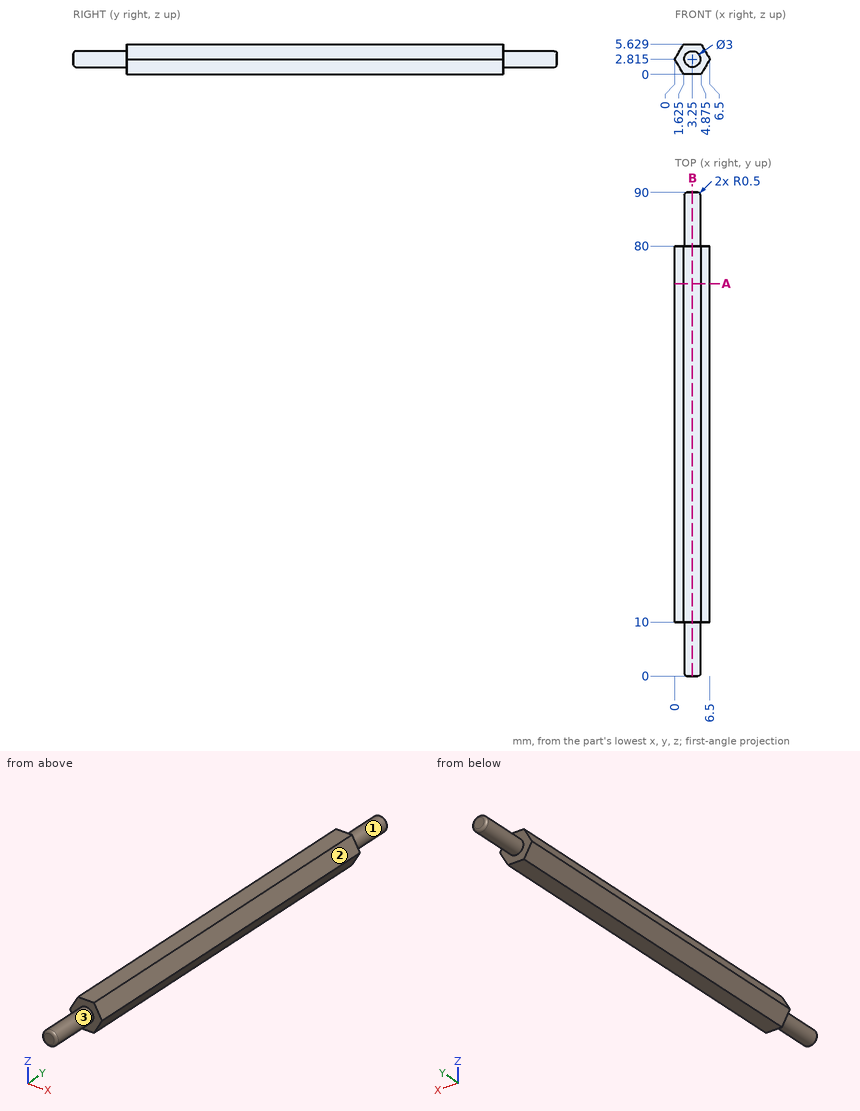
Geometry check sheet. Reference: drawing and pictorial views, mm from the part's lowest x, y, z. A direction names the side the tool comes from. Round coordinates to 2 decimals unless told otherwise and drop trailing zeros. Order: outer loops, then holes, each group sorted by start corner. A loop starts at its lowest first (then second) coordinate and runs counter-clockwise, first axis right, second up. Notation, with made-up numbers: (-11, 17.25) - (11, 17.25) arc R5 cw to (11, 26.25) - close; hole circle Ø2 at (80, 31). An arc over 180 degrees is marked (long way). Use a Markdown table: item, result. Add a question column.
1) Section check B-B (x = 3.25). Record the cut outline in (y, z) (1 decimal).
2) Section check A-A (y = 73). Record the cut outline in (x, z) (1 decimal).
3) Set-up check for the marked faces 1, 2 and 3: record each of +Z, -Z, +X, -X, +Y, -Y from which the full face is reachable in a straight line by a thin tool's end or side.
4) Gauge pin test, flat end, axial feed: P1, Ø1, axis at y = 12, z = 5, coming from the -X side. Record the tip position at first contact, or that the pin passes through.
5) Thickness scan on line 1 along Y through (x, z) = (5.75, 3.9); line 2 along X through (y, z) = (64, 0.7); line 3 along Z through (x, y) = (0.75, 73.5) (1 decimal). Record the ranges inside material, lowest first.
Established:
| question | item | result |
|---|---|---|
| 1 | outline | (0, 1.8) arc R0.5 ccw to (0.5, 1.3) - (10, 1.3) - (10, 0) - (80, 0) - (80, 1.3) - (89.5, 1.3) arc R0.5 ccw to (90, 1.8) - (90, 3.8) arc R0.5 ccw to (89.5, 4.3) - (80, 4.3) - (80, 5.6) - (10, 5.6) - (10, 4.3) - (0.5, 4.3) arc R0.5 ccw to (0, 3.8) - close |
| 2 | outline | (0, 2.8) - (1.6, 0) - (4.9, 0) - (6.5, 2.8) - (4.9, 5.6) - (1.6, 5.6) - close |
| 3 | face 1 | +Y |
| 3 | face 2 | +Z, +X, +Y, -Y |
| 3 | face 3 | -Y |
| 4 | P1 | x = 0.97 |
| 5 | line 1 | 10 to 80 |
| 5 | line 2 | 1.22 to 5.28 |
| 5 | line 3 | 1.5 to 4.1 |
